Source: CAD feature listing. Evaluate the final solid. Frame: model axes, mm. Coordinates: 2 decimals unless noted, no trailing zeros. Order: outer loops, then holes, each group sorted by start corner. A loop starts at its lowest first (then second) coordinate and runs counter-clockwise, first axis right, second up.
```python
from build123d import *

# Parameters (mm, degrees)
SKETCH_1_R          = 1.7
EXTRUDE_1_DEPTH     = 12.5
FILLET_1_R          = 5
SKETCH_2_R          = 1.7
CUT_EXTRUDE_1_DEPTH = 14


with BuildPart() as part:
    # 草图1 → 凸台-拉伸1 (new body)
    with BuildSketch(Plane(origin=(0, 0, 0), x_dir=(1, 0, 0), z_dir=(0, 1, 0))):
        with BuildLine():
            Line((-12.98390417, -16.013064432), (-4.531538935, 2.113091309))
            ThreePointArc((-4.531538935, 2.113091309), (0, 5), (4.531538935, 2.113091309))
            Line((4.531538935, 2.113091309), (12.98390417, -16.013064432))
            Line((12.98390417, -16.013064432), (-12.98390417, -16.013064432))
        make_face()
        with Locations(Location((0, 0, 0), (0, 0, 270))):
            Circle(SKETCH_1_R, mode=Mode.SUBTRACT)
    extrude(amount=EXTRUDE_1_DEPTH)

    # 圆角1
    fillet_1_edges = [part.edges().sort_by_distance(p)[0] for p in [
        (-12.98390417, 6.25, 16.013064432),
        (12.98390417, 6.25, 16.013064432),
    ]]
    fillet(fillet_1_edges, radius=FILLET_1_R)

    # 草图2 → 切除-拉伸1 (cut)
    with BuildSketch(Plane(origin=(0, 12.5, 0), x_dir=(1, 0, 0), z_dir=(0, 1, 0))):
        with Locations(Location((-5.135476284, -11.013064432, 0), (0, 0, 270))):
            Circle(SKETCH_2_R)
        with Locations(Location((5.135476284, -11.013064432, 0), (0, 0, 270))):
            Circle(SKETCH_2_R)
    extrude(amount=-CUT_EXTRUDE_1_DEPTH, mode=Mode.SUBTRACT)


solid = part.part
```
Q1. Section query B-B on x = 0. Output: boundary loops of the cut face in (y, z), plus the area to 3 significant figures.
Solutions:
outline: (0, -5) - (12.5, -5) - (12.5, -1.7) - (0, -1.7) - close; (0, 1.7) - (12.5, 1.7) - (12.5, 16.01) - (0, 16.01) - close
area: 220 mm2
Q2. Material intervals for line 1 along X through (y, z) = (6.25, 11); line 2 along X through (y, z) = (3.75, 10); line 3 along Z through (x, y) = (-5.25, 5.75), sorted ascending.
Solutions:
line 1: x = -10.14 to -6.84, -3.44 to 3.44, 6.84 to 10.14
line 2: x = -10.03 to -6.5, -3.77 to 3.77, 6.5 to 10.03
line 3: z = -0.57 to 9.32, 12.71 to 16.01
Q3. Pin query (flat end, axial travel): P1, Ø1, axis at y = 7.5, z = 7, coming from the -X side; P2, Ø1, axis at x = -2, y = 5, coming from the -Z side. Return the tip coordinate at first contact, or that it passes through.
Solutions:
P1: stops at x = -9.01
P2: stops at z = -4.77
Q4. Section query D-D on z = 0. Output: boundary loops of the cut face in (x, y).
Solutions:
outline: (-5.52, 0) - (-1.7, 0) - (-1.7, 12.5) - (-5.52, 12.5) - close; (1.7, 0) - (5.52, 0) - (5.52, 12.5) - (1.7, 12.5) - close
Q5. Pull-direction query (X, two-part tool) for faces 1 (the cylindrical face through (9.314, 6.338, 13.759)), 2 (the flat face through (0, 12.5, 8)), 3 (the cylindrical face through (4.48, 6.34, 12.58)); classes: pulls with the +X half, pulls with the -X half, needs draft (parallel to the pull), parting line crosses it, or undercut.
Solutions:
face 1: pulls with the +X half
face 2: needs draft
face 3: undercut
Q6. Section query C-C on z = 11.25. Output: boundary loops of the cut face in (x, y), plus the area to 3 significant figures.
Solutions:
outline: (-10.13, 0) - (-6.82, 0) - (-6.82, 12.5) - (-10.13, 12.5) - close; (-3.45, 0) - (3.45, 0) - (3.45, 12.5) - (-3.45, 12.5) - close; (6.82, 0) - (10.13, 0) - (10.13, 12.5) - (6.82, 12.5) - close
area: 169 mm2
Q7. Section query A-A on y = 11.75. Output: boundary loops of the cut face in (x, z).
Solutions:
outline: (-9.67, 8.9) - (-4.53, -2.11) arc R5 ccw to (4.53, -2.11) - (9.67, 8.9) arc R5 ccw to (5.14, 16.01) - (-5.14, 16.01) arc R5 ccw to start; hole circle Ø3.4 at (-5.14, 11.01); hole circle Ø3.4 at (0, 0); hole circle Ø3.4 at (5.14, 11.01)
